Here's how the part is built. I have some questions about the finished solid (model axes, mm). A direction names the side the tool comes from. Give positions to 0.01 mm unless a question says otherwise; leave off trailing zeros. Loops run counter-clockwise (first coordinate to the right, second up) from the corner with the lowest first, then second, coordinate; pieces in that order, holes last. Notation, with made-up numbers: (2, 41) - (42, 41) arc R17 ccw to (42, 72) - close; hole circle Ø10 at (-33, 48). An arc over 180 degrees is marked (long way). Use a Markdown table: item, result.
from build123d import *

# Parameters (mm, degrees)
F1_DEPTH = 10
F2_R     = 5
F3_DEPTH = 2
F4_W     = 4
F4_H     = 5
F5_DEPTH = 2
F6_R     = 5
F7_DEPTH = 2
F8_R     = 1


with BuildPart() as f1:
    # F0 (on Front) → F1 (new body, symmetric)
    with BuildSketch(Plane.XZ):
        with BuildLine():
            Line((27, 0), (0, 0))
            Line((0, 0), (0, -2))
            Line((0, -2), (27, -2))
            ThreePointArc((27, -2), (30.535534, -0.535534), (32, 3))
            Line((32, 3), (32, 30))
            Line((32, 30), (30, 30))
            Line((30, 30), (30, 3))
            ThreePointArc((30, 3), (29.12132, 0.87868), (27, 0))
        make_face()
    extrude(amount=F1_DEPTH, both=True)

    # F2 (on face) → F3 (cut, through all)
    with BuildSketch(Plane(origin=(30, 0, 0), x_dir=(0, -1, 0), z_dir=(-1, 0, 0))):
        with Locations((0, 20)):
            Circle(F2_R)
    extrude(amount=-F3_DEPTH, mode=Mode.SUBTRACT)

    # F4 (on face) → F5 (cut, through all)
    with BuildSketch(Plane(origin=(30, 0, 0), x_dir=(0, -1, 0), z_dir=(-1, 0, 0))):
        with Locations((8, 9.134532)):
            Rectangle(F4_W, F4_H)
    extrude(amount=-F5_DEPTH, mode=Mode.SUBTRACT)

    # F6 (on face) → F7 (cut, through all)
    with BuildSketch(Plane.XY):
        with Locations((10, 0)):
            Circle(F6_R)
    extrude(amount=-F7_DEPTH, mode=Mode.SUBTRACT)

    # F8
    f8_edges = [f1.edges().sort_by_distance(p)[0] for p in [
        (31, 10, 30),
        (31, -10, 30),
        (0, 10, -1),
        (0, -10, -1),
    ]]
    fillet(f8_edges, radius=F8_R)


solid = f1.part
(1) Suppose I cut it at C-C on x = 12.5. Write out the boundary of the cut face in (y, z), plus the area to 3 significant figures.
A:
| item | result |
|---|---|
| outline | (-10, -2) - (-4.33, -2) - (-4.33, 0) - (-10, 0) - close; (4.33, -2) - (10, -2) - (10, 0) - (4.33, 0) - close |
| area | 22.7 mm2 |
(2) Suppose I cut it at D-D on y = 0. Write out the boundary of the cut face in (x, z), plus the area to 3 significant figures.
A:
| item | result |
|---|---|
| outline | (0, -2) - (5, -2) - (5, 0) - (0, 0) - close; (15, -2) - (27, -2) arc R5 ccw to (32, 3) - (32, 15) - (30, 15) - (30, 3) arc R3 cw to (27, 0) - (15, 0) - close; (30, 25) - (32, 25) - (32, 30) - (30, 30) - close |
| area | 80.6 mm2 |
(3) If I drill on line 1 (Y direction, x = 10, z = -0.4); line 2 (X direction, y = 8.5, z = 11); line 3 (Z direction, x = 12.5, y = 6.5), over which ranges is the centre line in solid material (lowest first)?
A:
| item | result |
|---|---|
| line 1 | -10 to -5, 5 to 10 |
| line 2 | 30 to 32 |
| line 3 | -2 to 0 |
(4) Will these pins go through, and if not, where does the flat tip stop? pin 1 (6 mm diameter, centred on y = 5, z = 16, fed in from -X); pin 2 (0.6 mm diameter, centred on x = 31.5, y = -7, fed in from -Z); pin 3 (10 mm diameter, centred on x = 24.5, y = -6, fed in from +Z); pin 4 (8 mm diameter, centred on y = 0, z = 20, fed in from -X).
A:
| item | result |
|---|---|
| pin 1 | x = 30 |
| pin 2 | z = 0.29 |
| pin 3 | z = 1.34 |
| pin 4 | through |
(5) Suppose I cut it at A-A on y = -6.5. Write out the boundary of the cut face in (x, z), plus the area to 3 significant figures.
A:
| item | result |
|---|---|
| outline | (0, -2) - (27, -2) arc R5 ccw to (32, 3) - (32, 6.63) - (30, 6.63) - (30, 3) arc R3 cw to (27, 0) - (0, 0) - close; (30, 11.63) - (32, 11.63) - (32, 30) - (30, 30) - close |
| area | 111 mm2 |
(6) We'd pull the mould along Z, two halves only. Please class faces 1 (the face through (31, -6, 9)), 2 (the face through (30, 0, -1)), 3 (the face through (29.14, -0.14, 0.9)), 4 (the face through (31, -10, 20)): pulls with the +Z half, pulls with the -Z half, needs draft (parallel to the pull), parting line crosses it, or undercut.
A:
| item | result |
|---|---|
| face 1 | undercut |
| face 2 | pulls with the -Z half |
| face 3 | pulls with the +Z half |
| face 4 | needs draft |
(7) On a 3-axis mill with a long thin cutter (end or side, diameter ignored), from which of +Z, -Z, +X, -X, +Y, -Y can I reach the whole of each face in a straight line? I mean faces 5 (the face through (31, -8, 6.635)), 6 (the face through (30, 0, 14)), 7 (the face through (23.3, 10, -0.2)). Say none if no direction works.
A:
| item | result |
|---|---|
| face 5 | +X, -X, -Y |
| face 6 | +Z, -X, +Y, -Y |
| face 7 | +Z, -Z, +X, -X, +Y |
(8) Suppose I cut it at B-B on z = 20. Write out the boundary of the cut face in (x, y), plus the area to 3 significant figures.
A:
| item | result |
|---|---|
| outline | (30, -10) - (32, -10) - (32, -5) - (30, -5) - close; (30, 5) - (32, 5) - (32, 10) - (30, 10) - close |
| area | 20.0 mm2 |
